```python
from build123d import *

# Parameters (mm, degrees)
SKETCH2_W                    = 57.15
SKETCH2_H                    = 34.925
BASE_FLANGE1_DEPTH           = 3.175
EDGE_FLANGE1_STRIP_W         = 14.7
EDGE_FLANGE1_STRIP_H         = 3.175
EDGE_FLANGE1_STRIP_CUT_DEPTH = 34.925
EDGE_FLANGE1_DEPTH           = 34.925
CUT_EXTRUDE1_DEPTH           = 3.175
M6_CLEARANCE_HOLE1_D         = 6.6


# Sheet-metal steps are written as plain solids
with BuildPart() as part:
    # Sketch2 → Base-Flange1 (new body)
    with BuildSketch(Plane.XY):
        Rectangle(SKETCH2_W, SKETCH2_H)
    extrude(amount=BASE_FLANGE1_DEPTH)

    # Edge-Flange1 strip (across the edge) → Edge-Flange1 strip cut (cut)
    with BuildSketch(Plane(origin=(28.575, -17.4625, 3.175), x_dir=(-1, 0, 0), z_dir=(0, 1, 0))):
        with Locations((-6.35, -1.5875)):
            Rectangle(EDGE_FLANGE1_STRIP_W, EDGE_FLANGE1_STRIP_H)
    edge_flange1_strip_cut = extrude(amount=EDGE_FLANGE1_STRIP_CUT_DEPTH, mode=Mode.SUBTRACT)

    # Edge-Flange1 section (across the edge) → Edge-Flange1 (add)
    with BuildSketch(Plane(origin=(28.575, -17.4625, 3.175), x_dir=(-1, 0, 0), z_dir=(0, 1, 0))):
        with BuildLine():
            Line((-3.175, 1), (-3.175, 44.45))
            Line((-3.175, 44.45), (0, 44.45))
            Line((0, 44.45), (0, 1))
            ThreePointArc((0, 1), (0.292893219, 0.292893219), (1, 0))
            Line((1, 0), (1, -3.175))
            ThreePointArc((1, -3.175), (-1.952170811, -1.952170811), (-3.175, 1))
        make_face()
    edge_flange1 = extrude(amount=EDGE_FLANGE1_DEPTH)

    # Sketch10 → Cut-Extrude1 (cut)
    with BuildSketch(Plane(origin=(31.75, 0, 0), x_dir=(0, 0, -1), z_dir=(1, 0, 0))):
        Polygon((-4.175, 17.4625), (-47.625, -17.4625), (-47.625, 17.4625), align=None)
    cut_extrude1 = extrude(amount=-CUT_EXTRUDE1_DEPTH, mode=Mode.SUBTRACT)

    # Mirror1: Edge-Flange1 strip cut, Edge-Flange1, Cut-Extrude1 across plane
    add(edge_flange1_strip_cut.mirror(Plane(origin=(0, 0, 0), x_dir=(0, 0, 1), z_dir=(1, 0, 0))), mode=Mode.SUBTRACT)
    add(edge_flange1.mirror(Plane(origin=(0, 0, 0), x_dir=(0, 0, 1), z_dir=(1, 0, 0))))
    add(cut_extrude1.mirror(Plane(origin=(0, 0, 0), x_dir=(0, 0, 1), z_dir=(1, 0, 0))), mode=Mode.SUBTRACT)

    # M6 Clearance Hole1 (through all)
    with Locations(Plane.XY.offset(3.175)):
        with Locations((0, 0)):
            Hole(M6_CLEARANCE_HOLE1_D / 2)


solid = part.part
```
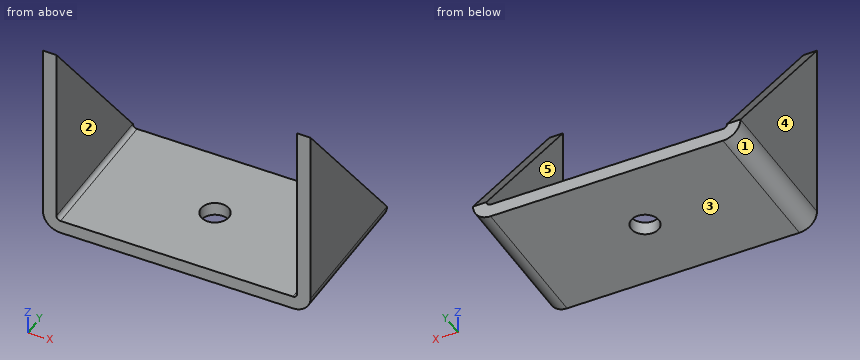
Read the model definition and answer for the solid it produces. Units are mm, in the model's axes. Face numbers are marked on the shaded views. A direction names the side the tool comes from. Coordinates: 2 decimals unless noted, no trailing zeros. Loops run counter-clockwise (first coordinate to the right, second up) from the corner with the lowest first, then second, coordinate; pieces in that order, holes last. Notation, with made-up numbers: (-15.5, 44.5) -> (11.5, 44.5) arc R13 cw to (11.5, 53.5) -> close; hole circle Ø5 at (56, -22.75). An arc over 180 degrees is marked (long way). Return JSON: item names as keys, results as strings.
Item 1: For the marked faces 4 and 5, determine the directions among +Z, -Z, +X, -X, +Y, -Y from which every point of the face is accessible in a straight line to the end or side of a thin tool.
Answers:
{"face 4": "+Z, -Z, -X, +Y, -Y", "face 5": "+Z, +Y, -Y"}
Item 2: Find section B-B (x = 0). Determine the outline of the cut face in (y, z) (1 decimal), plus the area to 3 significant figures.
Answers:
{"outline": "(-17.5, 0) -> (-3.3, 0) -> (-3.3, 3.2) -> (-17.5, 3.2) -> close; (3.3, 0) -> (17.5, 0) -> (17.5, 3.2) -> (3.3, 3.2) -> close", "area": "89.9 mm2"}
Item 3: Find section A-A (y = 0). Determine the outline of the cut face in (x, z) (3 decimals), plus the area to 3 significant figures.
Answers:
{"outline": "(-31.75, 4.175) arc R4.175 ccw to (-27.575, 0) -> (-3.3, 0) -> (-3.3, 3.175) -> (-27.575, 3.175) arc R1 cw to (-28.575, 4.175) -> (-28.575, 25.9) -> (-31.75, 25.9) -> close; (3.3, 0) -> (27.575, 0) arc R4.175 ccw to (31.75, 4.175) -> (31.75, 25.9) -> (28.575, 25.9) -> (28.575, 4.175) arc R1 cw to (27.575, 3.175) -> (3.3, 3.175) -> close", "area": "318 mm2"}
Item 4: Find the intervals of material crossed by probe 1 along X at (y, z) = (-14, 8) (3 decimals); probe 2 along Y at (x, z) = (0, 2); probe 3 along Z at (x, y) = (17, 7.5) (3 decimals), in increasing order.
Answers:
{"probe 1": "x = -31.75 to -28.575, 28.575 to 31.75", "probe 2": "y = -17.46 to -3.3, 3.3 to 17.46", "probe 3": "z = 0 to 3.175"}
Item 5: For a pull along X with two mould halves and no side action, classify the marked faces 1, 2 and 3 as +X half, -X half, draft (parallel to the pull), parting line (faces both ways), or undercut.
Answers:
{"face 1": "-X half", "face 2": "undercut", "face 3": "draft"}
Item 6: A flat-ended cylindrical pin translates along its axis: P1, Ø10.5, axis at x = -9.5, y = -5, coming from the +Z side (3 decimals). Find the tip coordinate at first contact, or state that the pin passes through.
Answers:
{"P1": "stops at z = 3.175"}
Item 7: Find section D-D (y = -5). Determine the outline of the cut face in (x, z) (3 decimals).
Answers:
{"outline": "(-31.75, 4.175) arc R4.175 ccw to (-27.575, 0) -> (27.575, 0) arc R4.175 ccw to (31.75, 4.175) -> (31.75, 32.12) -> (28.575, 32.12) -> (28.575, 4.175) arc R1 cw to (27.575, 3.175) -> (-27.575, 3.175) arc R1 cw to (-28.575, 4.175) -> (-28.575, 32.12) -> (-31.75, 32.12) -> close"}
